from build123d import *

# Parameters (mm, degrees)
F0_R     = 5.0038
F0_R_2   = 2.0066
F1_DEPTH = 3.9878
F2_R     = 5.0038
F2_R_2   = 2.0066
F3_DEPTH = 6.35
F4_SIZE  = 1.27
F6_DEPTH = 7.0104


with BuildPart() as f1:
    # F0 (on Top) → F1 (new body)
    with BuildSketch(Plane.XY):
        Circle(F0_R)
        Circle(F0_R_2, mode=Mode.SUBTRACT)
    extrude(amount=F1_DEPTH)

    # F2 (on face) → F3 (join)
    with BuildSketch(Plane.XY.offset(3.9878)):
        Polygon((-2.8575, -6.898615), (2.8575, -6.898615), (6.898615, -2.8575), (6.898615, 2.8575), (2.8575, 6.898615), (-2.8575, 6.898615), (-6.898615, 2.8575), (-6.898615, -2.8575), align=None)
        Circle(F2_R, mode=Mode.SUBTRACT)
        Circle(F2_R)
        Circle(F2_R_2, mode=Mode.SUBTRACT)
    extrude(amount=F3_DEPTH)

    # F4
    f4_edges = [f1.edges().sort_by_distance(p)[0] for p in [
        (-6.898615, 0, 10.3378),
        (-4.878058, 4.878058, 10.3378),
        (0, 6.898615, 10.3378),
        (4.878058, 4.878058, 10.3378),
        (6.898615, 0, 10.3378),
        (4.878058, -4.878058, 10.3378),
        (0, -6.898615, 10.3378),
        (-4.878058, -4.878058, 10.3378),
        (0, -6.898615, 3.9878),
        (-4.878058, -4.878058, 3.9878),
        (4.878058, -4.878058, 3.9878),
        (-6.898615, 0, 3.9878),
        (6.898615, 0, 3.9878),
        (4.878058, 4.878058, 3.9878),
        (0, 6.898615, 3.9878),
        (-4.878058, 4.878058, 3.9878),
    ]]
    chamfer(f4_edges, length=F4_SIZE)

    # F5 (on face) → F6 (cut)
    with BuildSketch(Plane.XY.offset(10.3378)):
        Polygon((1.9304, -3.343551), (3.8608, 0), (1.9304, 3.343551), (-1.9304, 3.343551), (-3.8608, 0), (-1.9304, -3.343551), align=None)
    extrude(amount=-F6_DEPTH, mode=Mode.SUBTRACT)


solid = f1.part
Can you work these out from the model? Positions are in its coordinate system, mm. A direction names the side the tool comes from. Round coordinates to 2 decimals unless told otherwise and drop trailing zeros. Order: outer loops, then holes, each group sorted by start corner. A loop starts at its lowest first (then second) coordinate and runs counter-clockwise, first axis right, second up. Notation, with made-up numbers: M 29.5,33.5 L 56.5,33.5 A35 cw 56.5,68.5 Z; hole C -12,38 d3. An arc over 180 degrees is marked long. Use a Markdown table: item, result.
1) I'm going to push flat-ended pins straight in: P1, Ø3, axis at x = 1, y = -1.5, coming from the +Z side; P2, Ø1.5, axis at y = -4.5, z = 8, coming from the -X side; P3, Ø2, axis at x = 0.5, y = 0.5, coming from the +Z side. Where does each tip first touch, or does it pass through?
Geometry says:
| item | result |
|---|---|
| P1 | stops at z = 3.33 |
| P2 | stops at x = -6.01 |
| P3 | passes through |
2) Imagine slicing it at B-B (z = 6.75). List the corners of the cut face in (x, y) for me.
Geometry says:
| item | result |
|---|---|
| outline | M -6.9,-2.86 L -2.86,-6.9 L 2.86,-6.9 L 6.9,-2.86 L 6.9,2.86 L 2.86,6.9 L -2.86,6.9 L -6.9,2.86 Z; hole M -3.86,0 L -1.93,-3.34 L 1.93,-3.34 L 3.86,0 L 1.93,3.34 L -1.93,3.34 Z |
3) If we mould it in two halves opening along Y, with no side actions, what happens to faces 1 (the face through (-4.85, 4.906, 7.136)), 2 (the face through (0, -3.344, 7)), 3 (the face through (-4.46, -4.41, 4.63))? For each: +Y half, -Y half, draft (parallel to the pull), parting line (faces both ways), or undercut.
Geometry says:
| item | result |
|---|---|
| face 1 | +Y half |
| face 2 | undercut |
| face 3 | -Y half |
4) Imagine slicing it at C-C (y = 0.75). List the corners of the cut face in (x, z) for me.
Geometry says:
| item | result |
|---|---|
| outline | M -6.9,5.26 L -5.63,3.99 L -4.95,3.99 L -4.95,0 L -1.86,0 L -1.86,3.33 L -3.43,3.33 L -3.43,10.34 L -5.63,10.34 L -6.9,9.07 Z; M 1.86,0 L 4.95,0 L 4.95,3.99 L 5.63,3.99 L 6.9,5.26 L 6.9,9.07 L 5.63,10.34 L 3.43,10.34 L 3.43,3.33 L 1.86,3.33 Z |
5) Imagine slicing it at D-D (y = -5.25). List the corners of the cut face in (x, z) for me.
Geometry says:
| item | result |
|---|---|
| outline | M -4.51,5.26 L -2.71,3.99 L 2.71,3.99 L 4.51,5.26 L 4.51,9.07 L 2.71,10.34 L -2.71,10.34 L -4.51,9.07 Z |
6) On a 3-axis mill with a long thin cutter (end or side, diameter ignored), from which of +Z, -Z, +X, -X, +Y, -Y can I reach the whole of each face in a straight line? I mean faces 4 (the face through (2.91, 1.65, 6.88)), 5 (the face through (-6.25, 0.04, 4.61)), 6 (the face through (-3.971, -3.045, 1.966)). Say none if no direction works.
Geometry says:
| item | result |
|---|---|
| face 4 | +Z |
| face 5 | -Z, -X, +Y, -Y |
| face 6 | -Z |
7) Imagine slicing it at A-A (x = 0). List the corners of the cut face in (y, z) for me, then the cut area to 3 significant figures.
Geometry says:
| item | result |
|---|---|
| outline | M -6.9,5.26 L -5.63,3.99 L -5,3.99 L -5,0 L -2.01,0 L -2.01,3.33 L -3.34,3.33 L -3.34,10.34 L -5.63,10.34 L -6.9,9.07 Z; M 2.01,0 L 5,0 L 5,3.99 L 5.63,3.99 L 6.9,5.26 L 6.9,9.07 L 5.63,10.34 L 3.34,10.34 L 3.34,3.33 L 2.01,3.33 Z |
| area | 64.1 mm² |
8) If I drill on line 1 along Y through (x, z) = (0, 2.35); line 2 along Z through (x, y) = (-4.25, -2.75); line 3 along Y through (x, z) = (1.75, 6.5), over which ranges is the centre line in solid material (lowest first)?
Geometry says:
| item | result |
|---|---|
| line 1 | y = -5 to -2.01, 2.01 to 5 |
| line 2 | z = 3.99 to 10.34 |
| line 3 | y = -6.9 to -3.34, 3.34 to 6.9 |
